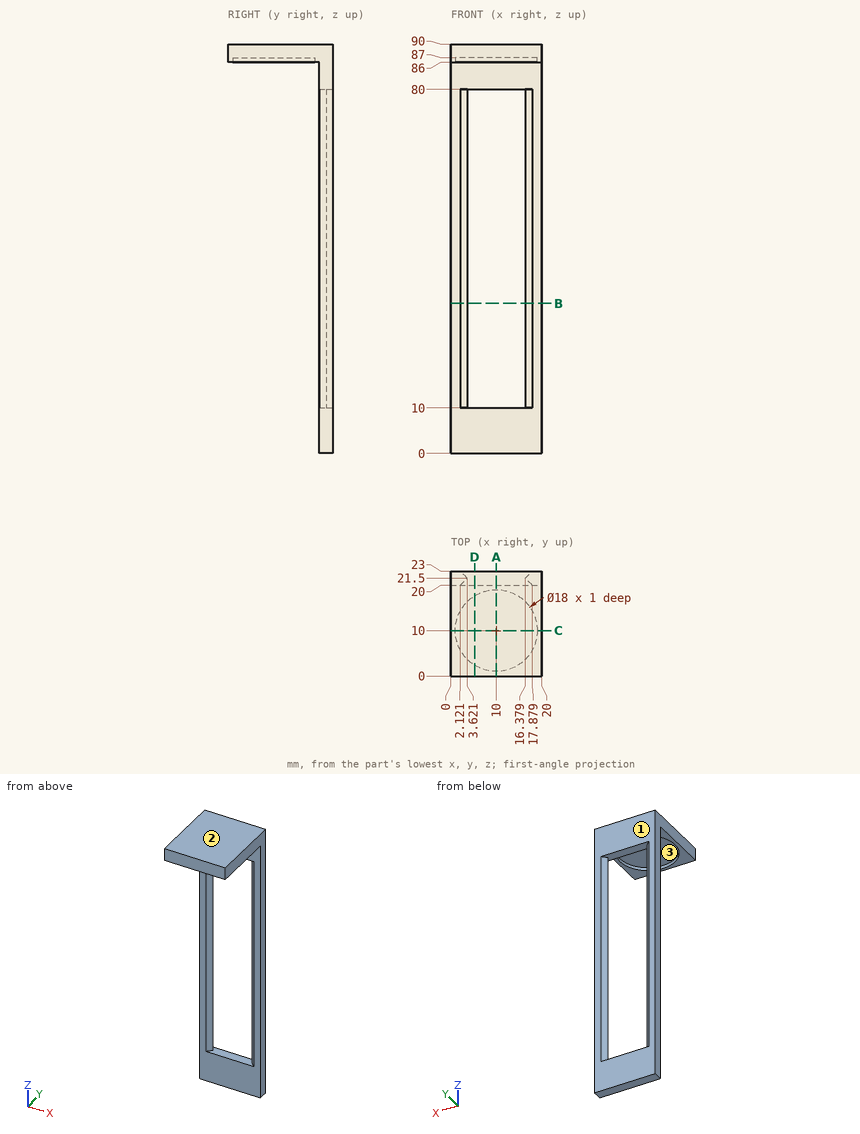
Here's the drawing with two shaded views (mm, measured from the low corner). I have some questions. Round coordinates to 2 decimals unless told otherwise and drop trailing zeros. Order: outer loops, then holes, each group sorted by start corner. A loop starts at its lowest first (then second) coordinate and runs counter-clockwise, first axis right, second up. Notation, with made-up numbers: (11, -14.75) -> (54, -14.75) arc R29 cw to (54, 14.25) -> close; hole circle Ø1 at (-20.5, 43.25). An arc over 180 degrees is marked (long way). Return JSON: item names as keys, results as strings.
Q1. For pin 1 Ø4 at (x, y) = (9, 6.5) entering from -Z; pin 2 Ø1.5 at (x, z) = (3, 55.5) entering from -Y, each with a flat end and sliding along its axis, tell me the tip position at first contact or that it passes through.
Filled sheet:
{"pin 1": "stops at z = 87", "pin 2": "stops at y = 20.13"}
Q2. I need wall thicknesses on line 1 along X through (y, z) = (10, 86.8); line 2 along Y through (x, z) = (10, 86.55); line 3 along Z through (x, y) = (11.5, 12). Which ranges of each line are inside material? Lowest first, please. Write a range as from..to.
Filled sheet:
{"line 1": "x = 0..1, 19..20", "line 2": "y = 0..1, 19..23", "line 3": "z = 87..90"}
Q3. If we section it at D-D on x = 5.25: List the corners of the cut face in (y, z) for me (1 decimal).
Filled sheet:
{"outline": "(0, 86) -> (2.4, 86) -> (2.4, 87) -> (17.6, 87) -> (17.6, 86) -> (20, 86) -> (20, 80) -> (23, 80) -> (23, 90) -> (0, 90) -> close; (20, 0) -> (23, 0) -> (23, 10) -> (20, 10) -> close"}
Q4. If we mould it in two halves opening along Y, with no side actions, what happens to the marked faces 1, 2 and 3? For each: released by +Y, released by -Y, zero draft, split by the parting line, or undercut.
Filled sheet:
{"face 1": "released by +Y", "face 2": "zero draft", "face 3": "undercut"}
Q5. If we section it at C-C on y = 10: List the corners of the cut face in (x, z) for me, plus the area to 3 significant figures.
Filled sheet:
{"outline": "(0, 86) -> (1, 86) -> (1, 87) -> (19, 87) -> (19, 86) -> (20, 86) -> (20, 90) -> (0, 90) -> close", "area": "62.0 mm^2"}
Q6. If we section it at B-B on z = 33: List the corners of the cut face in (x, y) for me, plus the area to 3 significant figures.
Filled sheet:
{"outline": "(0, 20) -> (2.12, 20) -> (3.62, 21.5) -> (2.12, 23) -> (0, 23) -> close; (16.38, 21.5) -> (17.88, 20) -> (20, 20) -> (20, 23) -> (17.88, 23) -> close", "area": "17.2 mm^2"}
Q7. If we section it at A-A on x = 10: List the corners of the cut face in (y, z) for me.
Filled sheet:
{"outline": "(0, 86) -> (1, 86) -> (1, 87) -> (19, 87) -> (19, 86) -> (20, 86) -> (20, 80) -> (23, 80) -> (23, 90) -> (0, 90) -> close; (20, 0) -> (23, 0) -> (23, 10) -> (20, 10) -> close"}
